Could you check a few things on this model? Use its own coordinates, in mm. Face numbers are marked on the shaded views. A direction names the side the tool comes from. Round coordinates to 2 decimals unless told otherwise and drop trailing zeros. Loops run counter-clockwise (first coordinate to the right, second up) from the corner with the lowest first, then second, coordinate; pieces in that order, holes last. Notation, with made-up numbers: (42.5, 59) -> (71.5, 59) arc R17 cw to (71.5, 64) -> close; hole circle Ø4 at (-8.75, 89.25). An arc over 180 degrees is marked (long way). Write each question's results on one line, items separated by ' | '. Start each with the question number.
1) Imagine slicing it at D-D, the plane y = 15. List the corners of the cut face in (x, z) for me, plus the area to 3 significant figures.
2) Imagine slicing it at C-C, the plane y = -7. List the corners of the cut face in (x, z) for me, plus the area to 3 significant figures.
3) Which directions (+Z, -Z, +X, -X, +Y, -Y) give clear straight access to the entire face, cutting with the end or side of a thin tool? Please do the marked faces 1, 2 and 3.
4) If I drill on probe 1 along Y at (x, z) = (0, 9.25); probe 2 along X at (y, z) = (-6.5, 17.25); probe 3 along X at (y, z) = (-17, 10), over which ranges is the centre line in solid material (lowest first)?
5) Imagine slicing it at B-B, the plane y = 0. List the corners of the cut face in (x, z) for me, plus the area to 3 significant figures.
6) We'd pull the mould along Y, two halves only. Please class the marked faces 4, 5 and 6: pulls with the +Y half, pulls with the -Y half, needs draft (parallel to the pull), parting line crosses it, or undercut.
7) For P1, Ø10, axis at y = 16, z = 6.5, coming from the -X side; P2, Ø4, axis at y = 5, z = 9, coming from the -X side; P3, Ø6, axis at y = 0, z = 3.5, coming from the -X side, each with a flat end and sliding along its axis, tell me the tip position at first contact or that it passes through.
8) Imagine slicing it at A-A, the plane x = 0. List the corners of the cut face in (y, z) for me, plus the area to 3 significant figures.
from build123d import *

# Parameters (mm, degrees)
F0_R     = 10
F1_DEPTH = 20


with BuildPart() as f1:
    # F0 (on Top) → F1 (new body)
    with BuildSketch(Plane.XY):
        with BuildLine():
            ThreePointArc((29.666667, -5.273097), (21.337731, -8.335878), (14.820652, -2.312633))
            ThreePointArc((14.820652, -2.312633), (14.5, 0), (14.820652, 2.312633))
            ThreePointArc((14.820652, 2.312633), (21.337731, 8.335878), (29.666667, 5.273097))
            ThreePointArc((29.666667, 5.273097), (30.220826, 5.780095), (30.822917, 6.229123))
            ThreePointArc((30.822917, 6.229123), (26.331077, 9.428888), (20.826087, 9.760845))
            ThreePointArc((20.826087, 9.760845), (19.841569, 11.632375), (18.68932, 13.405571))
            ThreePointArc((18.68932, 13.405571), (21.005287, 17.944736), (20.783802, 23.035774))
            ThreePointArc((20.783802, 23.035774), (20.073237, 22.792248), (19.341877, 22.621019))
            ThreePointArc((19.341877, 22.621019), (17.451033, 14.273836), (9.256765, 11.803063))
            ThreePointArc((9.256765, 11.803063), (7.082131, 12.652803), (5.220726, 14.062149))
            ThreePointArc((5.220726, 14.062149), (2.958081, 18.129936), (3.177151, 22.779502))
            ThreePointArc((3.177151, 22.779502), (2.417192, 22.87263), (1.654554, 22.940411))
            ThreePointArc((1.654554, 22.940411), (0, 23), (-1.654554, 22.940411))
            ThreePointArc((-1.654554, 22.940411), (-4.972729, 27.867393), (-10.500123, 30.043018))
            ThreePointArc((-10.500123, 30.043018), (-10.533434, 29.292619), (-10.641636, 28.549316))
            ThreePointArc((-10.641636, 28.549316), (-3.272802, 23.048837), (-5.220726, 14.062149))
            ThreePointArc((-5.220726, 14.062149), (-7.082131, 12.652803), (-9.256765, 11.803063))
            ThreePointArc((-9.256765, 11.803063), (-17.451033, 14.273836), (-19.341877, 22.621019))
            ThreePointArc((-19.341877, 22.621019), (-20.073237, 22.792248), (-20.783802, 23.035774))
            ThreePointArc((-20.783802, 23.035774), (-21.005287, 17.944736), (-18.68932, 13.405571))
            ThreePointArc((-18.68932, 13.405571), (-19.841569, 11.632375), (-20.826087, 9.760845))
            ThreePointArc((-20.826087, 9.760845), (-26.331077, 9.428888), (-30.822917, 6.229123))
            ThreePointArc((-30.822917, 6.229123), (-30.220826, 5.780095), (-29.666667, 5.273097))
            ThreePointArc((-29.666667, 5.273097), (-21.337731, 8.335878), (-14.820652, 2.312633))
            ThreePointArc((-14.820652, 2.312633), (-14.5, 0), (-14.820652, -2.312633))
            ThreePointArc((-14.820652, -2.312633), (-21.337731, -8.335878), (-29.666667, -5.273097))
            ThreePointArc((-29.666667, -5.273097), (-30.220826, -5.780095), (-30.822917, -6.229123))
            ThreePointArc((-30.822917, -6.229123), (-26.331077, -9.428888), (-20.826087, -9.760845))
            ThreePointArc((-20.826087, -9.760845), (-19.841569, -11.632375), (-18.68932, -13.405571))
            ThreePointArc((-18.68932, -13.405571), (-21.005287, -17.944736), (-20.783802, -23.035774))
            ThreePointArc((-20.783802, -23.035774), (-20.073237, -22.792248), (-19.341877, -22.621019))
            ThreePointArc((-19.341877, -22.621019), (-17.451033, -14.273836), (-9.256765, -11.803063))
            ThreePointArc((-9.256765, -11.803063), (-7.082131, -12.652803), (-5.220726, -14.062149))
            ThreePointArc((-5.220726, -14.062149), (-3.272802, -23.048837), (-10.641636, -28.549316))
            ThreePointArc((-10.641636, -28.549316), (-10.533434, -29.292619), (-10.500123, -30.043018))
            ThreePointArc((-10.500123, -30.043018), (-4.972729, -27.867393), (-1.654554, -22.940411))
            ThreePointArc((-1.654554, -22.940411), (0, -23), (1.654554, -22.940411))
            ThreePointArc((1.654554, -22.940411), (4.972729, -27.867393), (10.500123, -30.043018))
            ThreePointArc((10.500123, -30.043018), (10.533434, -29.292619), (10.641636, -28.549316))
            ThreePointArc((10.641636, -28.549316), (3.272802, -23.048837), (5.220726, -14.062149))
            ThreePointArc((5.220726, -14.062149), (7.082131, -12.652803), (9.256765, -11.803063))
            ThreePointArc((9.256765, -11.803063), (17.451033, -14.273836), (19.341877, -22.621019))
            ThreePointArc((19.341877, -22.621019), (20.073237, -22.792248), (20.783802, -23.035774))
            ThreePointArc((20.783802, -23.035774), (21.005287, -17.944736), (18.68932, -13.405571))
            ThreePointArc((18.68932, -13.405571), (19.841569, -11.632375), (20.826087, -9.760845))
            ThreePointArc((20.826087, -9.760845), (26.331077, -9.428888), (30.822917, -6.229123))
            ThreePointArc((30.822917, -6.229123), (30.220826, -5.780095), (29.666667, -5.273097))
        make_face()
        Circle(F0_R, mode=Mode.SUBTRACT)
        with BuildLine():
            ThreePointArc((1.654554, 22.940411), (2.417192, 22.87263), (3.177151, 22.779502))
            ThreePointArc((3.177151, 22.779502), (6.035405, 26.795099), (10.641636, 28.549316))
            ThreePointArc((10.641636, 28.549316), (10.533434, 29.292619), (10.500123, 30.043018))
            ThreePointArc((10.500123, 30.043018), (4.972729, 27.867393), (1.654554, 22.940411))
        make_face()
    extrude(amount=F1_DEPTH)


solid = f1.part
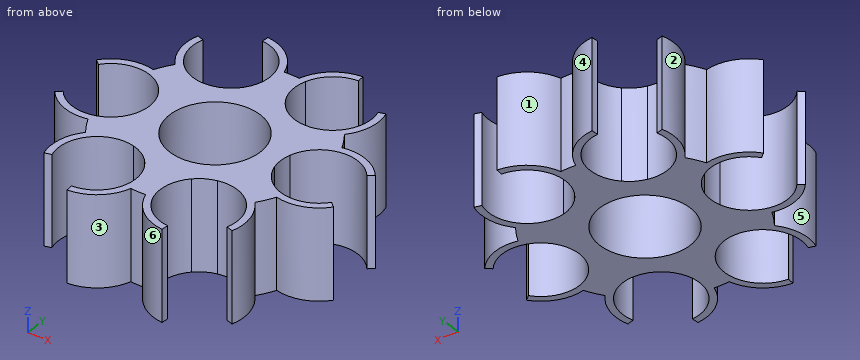
Checked values:
1) outline: (-19.85, 0) -> (-18.06, 0) -> (-18.06, 20) -> (-19.85, 20) -> close; (-4.41, 0) -> (4.41, 0) -> (4.41, 20) -> (-4.41, 20) -> close; (18.06, 0) -> (19.85, 0) -> (19.85, 20) -> (18.06, 20) -> close | area: 248 mm^2
2) outline: (-30.14, 0) -> (-27.82, 0) -> (-27.82, 20) -> (-30.14, 20) -> close; (-18.18, 0) -> (-7.14, 0) -> (-7.14, 20) -> (-18.18, 20) -> close; (7.14, 0) -> (18.18, 0) -> (18.18, 20) -> (7.14, 20) -> close; (27.82, 0) -> (30.14, 0) -> (30.14, 20) -> (27.82, 20) -> close | area: 534 mm^2
3) face 1: +Z, -Z, +Y | face 2: +Z, -Z, -X | face 3: +Z, -Z, -Y
4) probe 1: -23 to -10, 10 to 23 | probe 2: -30.6 to -28.48, -17.52 to -7.6, 7.6 to 17.52, 28.48 to 30.6 | probe 3: -20.75 to -19.16, -3.31 to 3.31, 19.16 to 20.75
5) outline: (-14.5, 0) -> (-10, 0) -> (-10, 20) -> (-14.5, 20) -> close; (10, 0) -> (14.5, 0) -> (14.5, 20) -> (10, 20) -> close | area: 180 mm^2
6) face 4: pulls with the +Y half | face 5: undercut | face 6: pulls with the -Y half
7) P1: x = -21.23 | P2: x = -30.82 | P3: x = -15.05
8) outline: (-23, 0) -> (-10, 0) -> (-10, 20) -> (-23, 20) -> close; (10, 0) -> (23, 0) -> (23, 20) -> (10, 20) -> close | area: 520 mm^2
